The figure shows three views and two pictorial views of one solid part (mm, origin at its lowest corner). Answer the questions. A direction names the side the tool comes from. Coordinates: 2 decimals unless noted, no trailing zeros. Loops run counter-clockwise (first coordinate to the right, second up) from the corner with the lowest first, then second, coordinate; pieces in that order, holes last. Notation, with made-up numbers: (44, 45) - (91, 45) arc R12 ccw to (91, 58) - close; hole circle Ø1 at (55, 67). An arc over 180 degrees is marked (long way). Write each question's results on one line, items separated by ' | '. Start each with the question number.
Item 1: Section A-A, the plane y = 11 is taken. Write down the section's boundary in (x, z).
Item 2: For a pull along X with two mould halves and no side action, classify the marked faces 1, 2 and 3 as +X half, -X half, draft (parallel to the pull), parting line (faces both ways), or undercut.
Item 3: Section C-C, the plane z = 9 is taken. Write down the section's boundary in (x, y).
Item 4: Each of these flat-tipped pins is pushed along its axis until it touches: pin 1 Ø2 at (x, z) = (4, 4.5) entering from -Y; pin 2 Ø3 at (x, y) = (7, 11) entering from +Z. Where does it stop, or does it pass through?
Item 5: Section B-B, the plane x = 7 is taken. Write down the section's boundary in (y, z).
Item 6: Consider probe 1 along X at (y, z) = (2, 3.5); probe 2 along X at (y, z) = (5, 6.75); probe 3 along Y at (x, z) = (15, 4.75). Determine where each line is inside the solid, lowest interval first. Write a range as [from, to].
Item 7: Section D-D, the plane x = 4 is taken. Write down the section's boundary in (y, z), plus the area to 3 significant figures.
Item 8: A tool of negligible diameter and unlimited length cuts with its end or side. For the marked faces 4 and 5, from which of +Z, -Z, +X, -X, +Y, -Y can it reach the whole face along a straight path? Write none if from no direction.
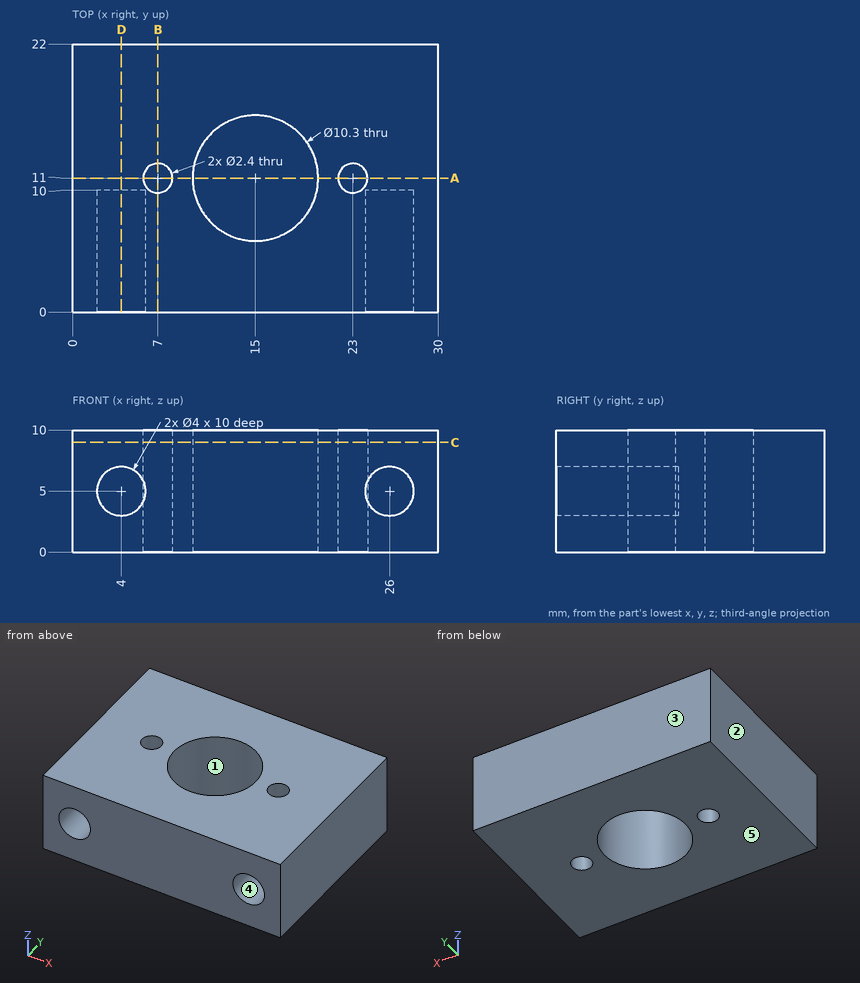
Answer key:
1) outline: (0, 0) - (5.8, 0) - (5.8, 10) - (0, 10) - close; (8.2, 0) - (9.85, 0) - (9.85, 10) - (8.2, 10) - close; (20.15, 0) - (21.8, 0) - (21.8, 10) - (20.15, 10) - close; (24.2, 0) - (30, 0) - (30, 10) - (24.2, 10) - close
2) face 1: undercut | face 2: -X half | face 3: draft
3) outline: (0, 0) - (30, 0) - (30, 22) - (0, 22) - close; hole circle Ø2.4 at (7, 11); hole circle Ø10.3 at (15, 11); hole circle Ø2.4 at (23, 11)
4) pin 1: stops at y = 10 | pin 2: stops at z = 10
5) outline: (0, 0) - (9.8, 0) - (9.8, 10) - (0, 10) - close; (12.2, 0) - (22, 0) - (22, 10) - (12.2, 10) - close
6) probe 1: x = [0, 2.68], [5.32, 24.68], [27.32, 30] | probe 2: x = [0, 3.03], [4.97, 25.03], [26.97, 30] | probe 3: y = [0, 5.85], [16.15, 22]
7) outline: (0, 0) - (22, 0) - (22, 10) - (0, 10) - (0, 7) - (10, 7) - (10, 3) - (0, 3) - close | area: 180 mm^2
8) face 4: -Y | face 5: -Z, +X, -X, +Y, -Y
